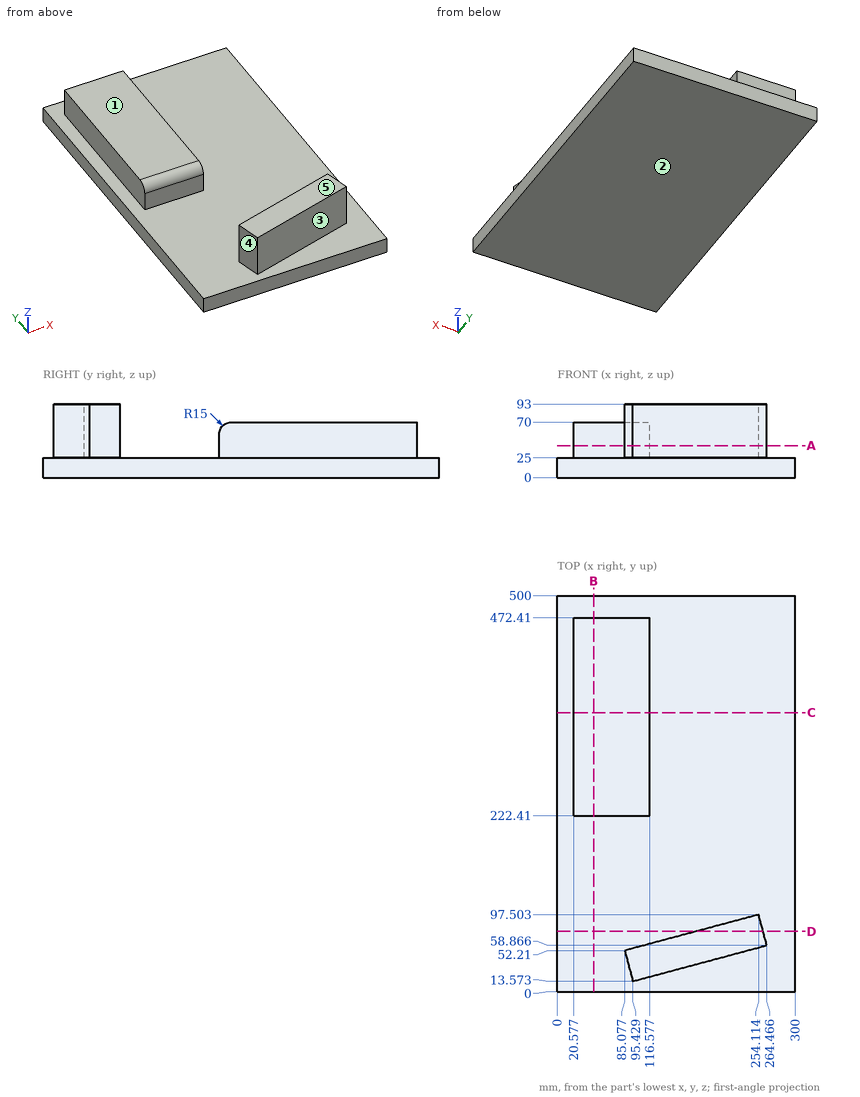
Geometry check sheet. Reference: drawing and pictorial views, mm from the part's lowest x, y, z. A direction names the side the tool comes from. Round coordinates to 2 decimals unless told otherwise and drop trailing zeros. Order: outer loops, then holes, each group sorted by start corner. A loop starts at its lowest first (then second) coordinate and runs counter-clockwise, first axis right, second up. Notation, with made-up numbers: (7, 9) - (11, 9) arc R13 ccw to (11, 27) - close; hole circle Ø10 at (-23, 68). An arc over 180 degrees is marked (long way). One line per question, with ' | ' between items. Start each with the question number.
(1) Access from +Z, -Z, +X, -X, +Y, -Y to the whole of each face (thin tool, end or side, straight path). Record for the marked faces 1 and 2.
(2) Sectioned sample at B-B on x = 46. Record the cut outline in (y, z), and give its area (3 significant figures).
(3) Sectioned sample at A-A on z = 40.5. Record the cut outline in (x, y), and give its area (3 significant figures).
(4) Sectioned sample at D-D on y = 76.5. Record the cut outline in (x, z), and give its area (3 significant figures).
(5) Sectioned sample at C-C on y = 352.5. Record the cut outline in (x, z), and give its area (3 significant figures).
(6) Depth check by flat-ended pin: pin 1 Ø12 at (y, z) = (401.5, 64) entering from -X; pin 2 Ø3 at (x, y) = (218, 177) entering from +Z; pin 3 Ø15 at (x, z) = (68, 37) entering from -Y. Enter the tip coordinate at first touch or a pass-through.
(7) Release check for a two-part mould opening along X. For the marked faces 3, 4 and 5 record: released by +X, released by -X, zero draft, split by the parting line, or undercut.
(8) Thickness scan on L1, parallel to X at y = 347.5, z = 58; L2, parallel to Z at x = 226, y = 126; L3, parallel to Z at x = 52.5, y = 355. Record the ranges inside material, lowest first. Write a range as [from, to].
Conclusion:
1) face 1: +Z, +X, -X, +Y | face 2: -Z, +X, -X, +Y, -Y
2) outline: (0, 0) - (500, 0) - (500, 25) - (472.41, 25) - (472.41, 70) - (237.41, 70) arc R15 ccw to (222.41, 55) - (222.41, 25) - (0, 25) - close | area: 23,700 mm2
3) outline: (20.58, 222.41) - (116.58, 222.41) - (116.58, 472.41) - (20.58, 472.41) - close; (85.08, 52.21) - (95.43, 13.57) - (264.47, 58.87) - (254.11, 97.5) - close | area: 31,000 mm2
4) outline: (0, 0) - (300, 0) - (300, 25) - (259.74, 25) - (259.74, 93) - (175.73, 93) - (175.73, 25) - (0, 25) - close | area: 13,200 mm2
5) outline: (0, 0) - (300, 0) - (300, 25) - (116.58, 25) - (116.58, 70) - (20.58, 70) - (20.58, 25) - (0, 25) - close | area: 11,800 mm2
6) pin 1: stops at x = 20.58 | pin 2: stops at z = 25 | pin 3: stops at y = 222.41
7) face 3: released by +X | face 4: released by -X | face 5: zero draft
8) L1: x = [20.58, 116.58] | L2: z = [0, 25] | L3: z = [0, 70]
